from build123d import *

# Parameters (mm, degrees)
SKETCH2_R           = 1
SKETCH2_W           = 2.12
SKETCH2_H           = 12.1
BOSS_EXTRUDE2_DEPTH = 2
BOSS_EXTRUDE3_DEPTH = 3
CHAMFER1_SIZE2      = 2
CHAMFER1_SIZE       = 5


with BuildPart() as part:
    # Sketch2 → Boss-Extrude2 (new body)
    with BuildSketch(Plane(origin=(0, 0, 0), x_dir=(1, 0, 0), z_dir=(0, 1, 0))):
        with BuildLine():
            Line((-10, 24.439438281), (-10, 17.439438281))
            Line((-10, 17.439438281), (10, 17.439438281))
            Line((10, 17.439438281), (10, 24.439438281))
            ThreePointArc((10, 24.439438281), (26.021613026, 19.342266443), (40, 10))
            Line((40, 10), (40, -10))
            Line((40, -10), (-40, -10))
            Line((-40, -10), (-40, 10))
            ThreePointArc((-40, 10), (-26.021613026, 19.342266443), (-10, 24.439438281))
        make_face()
        with Locations(Location((-37.490381057, -7.5, 0), (0, 0, 270))):
            Circle(SKETCH2_R, mode=Mode.SUBTRACT)
        with Locations(Location((37.490381057, -7.5, 0), (0, 0, 90))):
            Circle(SKETCH2_R, mode=Mode.SUBTRACT)
        with Locations(Location((-24.5, 15, 0), (0, 0, 270))):
            Circle(SKETCH2_R, mode=Mode.SUBTRACT)
        with Locations(Location((24.5, 15, 0), (0, 0, 90))):
            Circle(SKETCH2_R, mode=Mode.SUBTRACT)
        with Locations((15.56, 1.55)):
            Rectangle(SKETCH2_W, SKETCH2_H, mode=Mode.SUBTRACT)
        with Locations((-15.56, 1.55)):
            Rectangle(SKETCH2_W, SKETCH2_H, mode=Mode.SUBTRACT)
    extrude(amount=BOSS_EXTRUDE2_DEPTH)

    # Sketch3 → Boss-Extrude3 (add)
    with BuildSketch(Plane(origin=(0, 2, 0), x_dir=(1, 0, 0), z_dir=(0, 1, 0))):
        Polygon((12.419999998, -4.5), (37.42, -4.5), (37.42, 7.6), (12.419999998, 7.6), (12.419999998, 8.599999996), (38.419999998, 8.599999996), (38.419999998, -5.499999996), (12.419999998, -5.499999996), align=None)
        Polygon((-12.419999998, -4.5), (-12.419999998, -5.499999996), (-38.419999998, -5.499999996), (-38.419999998, 8.599999996), (-12.419999998, 8.599999996), (-12.419999998, 7.6), (-37.42, 7.6), (-37.42, -4.5), align=None)
    extrude(amount=BOSS_EXTRUDE3_DEPTH)

    # Chamfer1
    chamfer1_edges = [part.edges().sort_by_distance(p)[0] for p in [
        (0, 2, -17.439438281),
    ]]
    chamfer1_side = [part.faces().sort_by_distance(p)[0] for p in [
        (0, 2, -17.399438281),
    ]]
    chamfer(chamfer1_edges, length=CHAMFER1_SIZE - 0.0001, length2=CHAMFER1_SIZE2 - 0.0001, reference=chamfer1_side[0])  # a hair under: the kernel refuses the full size


solid = part.part
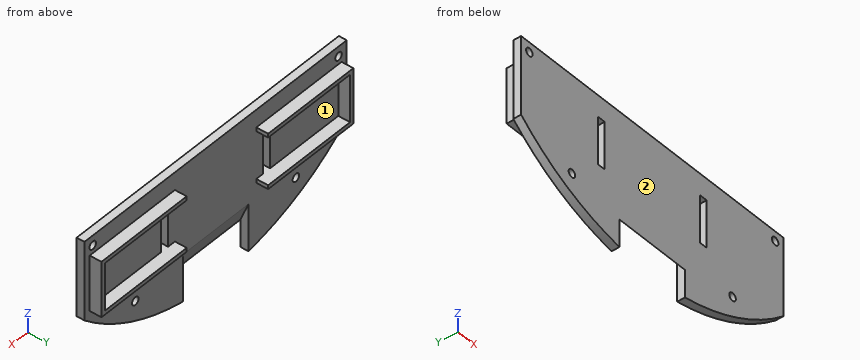
Source: CAD feature listing. Evaluate the final solid. Frame: model axes, mm. Face numbers are marked on the shaded views. Round coordinates to 2 decimals unless told otherwise and drop trailing zeros. Loops run counter-clockwise (first coordinate to the right, second up) from the corner with the lowest first, then second, coordinate; pieces in that order, holes last. Notation, with made-up numbers: (43, 13.25) -> (83, 13.25) arc R21 ccw to (83, 20.25) -> close; hole circle Ø3 at (58.5, -29). An arc over 180 degrees is marked (long way). Answer as a JSON object with one key per item and string values. Group by question number.
Q1. Contact query for flat-ended pins moving along their axis: P1, Ø2, axis at y = 3.5, z = -10, coming from the -X side; P2, Ø1.6, axis at y = 1.5, z = -16.5, coming from the -X side; P3, Ø2.5, axis at x = 32, y = 4, coming from the -Z side; P4, Ø0.8, axis at y = 3.5, z = -8.5, coming from the +X side. Output: stop coordinate, or through.
Q2. Section query A-A (y = 3.6). Output: boundary loops of the cut face in (x, z), plus the area to 3 significant figures.
Q3. Section query C-C (x = 24.5). Output: boundary loops of the cut face in (y, z), plus the area to 3 significant figures.
Q4. Mould query, pull axis Z, two halves, no side actions, for the marked faces 1 and 2. Classes: pulls with the +Z half, pulls with the -Z half, needs draft (parallel to the pull), parting line crosses it, or undercut.
Q5. Ray query, line 1 (X direction, y = 1.4, z = 7.5); line 2 (X direction, y = 2.35, z = -5.5); line 3 (Z direction, x = -26, y = 3.05). Return the intervals inside material, ascending. Write a range as from..to.
Q6. Section query B-B (z = 7.5). Output: boundary loops of the cut face in (x, y).
Completed:
{
 "1": {"P1": "through", "P2": "x = -32.52", "P3": "z = -8.6", "P4": "x = 38.42"},
 "2": {"outline": "(-38.42, -8.6) -> (-12.42, -8.6) -> (-12.42, -7.6) -> (-37.42, -7.6) -> (-37.42, 4.5) -> (-12.42, 4.5) -> (-12.42, 5.5) -> (-38.42, 5.5) -> close; (12.42, -8.6) -> (38.42, -8.6) -> (38.42, 5.5) -> (12.42, 5.5) -> (12.42, 4.5) -> (37.42, 4.5) -> (37.42, -7.6) -> (12.42, -7.6) -> close", "area": "128 mm²"},
 "3": {"outline": "(0, -20.05) -> (2, -20.05) -> (2, -16) -> (0, -16) -> close; (0, -14) -> (2, -14) -> (2, -8.6) -> (5, -8.6) -> (5, -7.6) -> (2, -7.6) -> (2, 4.5) -> (5, 4.5) -> (5, 5.5) -> (2, 5.5) -> (2, 10) -> (0, 10) -> close", "area": "62.1 mm²"},
 "4": {"face 1": "undercut", "face 2": "needs draft"},
 "5": {"line 1": "-40..-38.49, -36.49..36.49, 38.49..40", "line 2": "-38.42..-37.42, 37.42..38.42", "line 3": "-8.6..-7.6, 4.5..5.5"},
 "6": {"outline": "(-40, 0) -> (-38.49, 0) -> (-38.49, 2) -> (-40, 2) -> close; (-36.49, 0) -> (36.49, 0) -> (36.49, 2) -> (-36.49, 2) -> close; (38.49, 0) -> (40, 0) -> (40, 2) -> (38.49, 2) -> close"}
}
